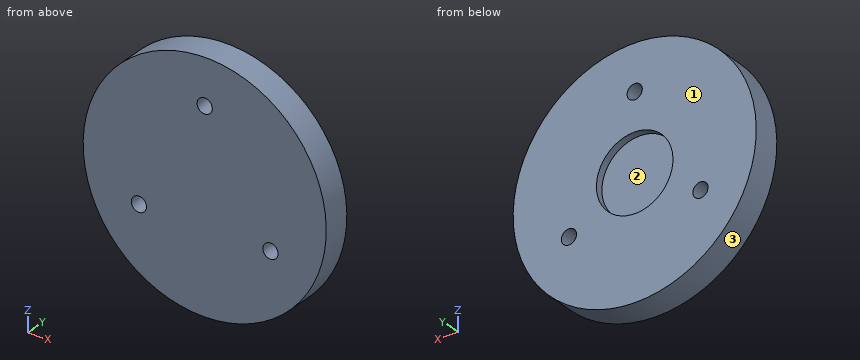
from build123d import *

# Parameters (mm, degrees)
SKETCH1_R           = 50.8
BOSS_EXTRUDE1_DEPTH = 11.9888
SKETCH3_R           = 3.175
CUT_EXTRUDE1_DEPTH  = 73.835508685
CIRPATTERN1_COUNT   = 3
SKETCH4_R           = 16.002
CUT_EXTRUDE2_DEPTH  = 3.175


with BuildPart() as part:
    # Sketch1 → Boss-Extrude1 (new body)
    with BuildSketch(Plane(origin=(0, 0, 0), x_dir=(1, 0, 0), z_dir=(0, 1, 0))):
        with Locations(Location((0, 0, 0), (0, 0, 90))):
            Circle(SKETCH1_R)
    extrude(amount=BOSS_EXTRUDE1_DEPTH)

    # Sketch3 → Cut-Extrude1 (cut, through all)
    with BuildSketch(Plane.XZ):
        with Locations(Location((0, 31.75, 0), (0, 0, 270))):
            Circle(SKETCH3_R)
    cut_extrude1 = extrude(amount=-CUT_EXTRUDE1_DEPTH, mode=Mode.SUBTRACT)

    # CirPattern1: Cut-Extrude1 ×3 about axis
    cirpattern1_axis = Axis((0, 0, 0), (0, 1, 0))
    for i in range(1, CIRPATTERN1_COUNT):
        add(cut_extrude1.rotate(cirpattern1_axis, i * 360 / CIRPATTERN1_COUNT), mode=Mode.SUBTRACT)

    # Sketch4 → Cut-Extrude2 (cut)
    with BuildSketch(Plane(origin=(0, 11.9888, 0), x_dir=(1, 0, 0), z_dir=(0, 1, 0))):
        with Locations(Location((0, 0, 0), (0, 0, 270))):
            Circle(SKETCH4_R)
    extrude(amount=-CUT_EXTRUDE2_DEPTH, mode=Mode.SUBTRACT)


solid = part.part
Source: CAD feature listing. Evaluate the final solid. Frame: model axes, mm. Face numbers are marked on the shaded views. Round coordinates to 2 decimals unless told otherwise and drop trailing zeros. Loops run counter-clockwise (first coordinate to the right, second up) from the corner with the lowest first, then second, coordinate; pieces in that order, holes last. Notation, with made-up numbers: M 31.25,27.25 L 56.25,27.25 A24 ccw 56.25,54.25 Z; hole C 69,41.5 d8. An arc over 180 degrees is marked long. Return JSON: item names as keys, results as strings. Group by question number.
1. Pin query (flat end, axial travel): pin 1 (2 mm diameter, centred on x = 37.5, y = 10, fed in from +Z); pin 2 (12 mm diameter, centred on x = 4, z = -24.5, fed in from -Y); pin 3 (6 mm diameter, centred on x = 22, y = 4, fed in from +Z). Return the tip coordinate at first contact, or that it passes through.
2. Section query A-A on x = 0. Output: boundary loops of the cut face in (y, z) (3 decimals).
3. Material intervals for line 1 along X through (y, z) = (10.3, 0); line 2 along Z through (x, y) = (2.5, 7.75); line 3 along Z through (x, y) = (-30, 5.5), sorted ascending. Write a range as from..to.
4. Section query D-D on x = -10.5. Output: boundary loops of the cut face in (y, z), and give its area (3 significant figures).
5. Mould query, pull axis X, two halves, no side actions, for the marked faces 1, 2 and 3. Classes: released by +X, released by -X, zero draft, split by the parting line, or undercut.
6. Section query B-B on z = 0. Output: boundary loops of the cut face in (x, y), and give its area (3 significant figures).
7. Section query C-C on z = 32. Output: boundary loops of the cut face in (x, y).
Checks:
{
 "1": {"pin 1": "stops at z = 35.33", "pin 2": "stops at y = 0", "pin 3": "stops at z = 47.11"},
 "2": {"outline": "M 0,-50.8 L 11.989,-50.8 L 11.989,-16.002 L 8.814,-16.002 L 8.814,16.002 L 11.989,16.002 L 11.989,28.575 L 0,28.575 Z; M 0,34.925 L 11.989,34.925 L 11.989,50.8 L 0,50.8 Z"},
 "3": {"line 1": "x = -50.8..-16, 16..50.8", "line 2": "z = -50.74..29.79, 33.71..50.74", "line 3": "z = -41..-17.83, -13.92..41"},
 "4": {"outline": "M 0,-49.7 L 11.99,-49.7 L 11.99,-12.08 L 8.81,-12.08 L 8.81,12.08 L 11.99,12.08 L 11.99,49.7 L 0,49.7 Z", "area": "1,120 mm²"},
 "5": {"face 1": "zero draft", "face 2": "undercut", "face 3": "split by the parting line"},
 "6": {"outline": "M -50.8,0 L 50.8,0 L 50.8,11.99 L 16,11.99 L 16,8.81 L -16,8.81 L -16,11.99 L -50.8,11.99 Z", "area": "1,120 mm²"},
 "7": {"outline": "M -39.45,0 L -3.17,0 L -3.17,11.99 L -39.45,11.99 Z; M 3.17,0 L 39.45,0 L 39.45,11.99 L 3.17,11.99 Z"}
}
